```python
from build123d import *

# Parameters (mm, degrees)
SKETCH1_R           = 86.9315
BOSS_EXTRUDE1_DEPTH = 2.54
SKETCH2_W           = 104.14
SKETCH2_H           = 104.14
CUT_EXTRUDE1_DEPTH  = 2.54
SKETCH3_R           = 9.525
SKETCH3_W           = 104.14
SKETCH3_H           = 104.14
CUT_EXTRUDE3_DEPTH  = 203.2


with BuildPart() as part:
    # Sketch1 → Boss-Extrude1 (new body)
    with BuildSketch(Plane(origin=(0, 0, 0), x_dir=(1, 0, 0), z_dir=(0, 1, 0))):
        with Locations(Location((0, 0, 0), (0, 0, 270))):
            Circle(SKETCH1_R)
    extrude(amount=BOSS_EXTRUDE1_DEPTH)

    # Sketch2 → Cut-Extrude1 (cut)
    with BuildSketch(Plane(origin=(0, 2.54, 0), x_dir=(1, 0, 0), z_dir=(0, 1, 0))):
        Rectangle(SKETCH2_W, SKETCH2_H)
    extrude(amount=-CUT_EXTRUDE1_DEPTH, mode=Mode.SUBTRACT)

    # Sketch3 → Cut-Extrude3 (cut)
    with BuildSketch(Plane(origin=(0, 2.54, 0), x_dir=(1, 0, 0), z_dir=(0, 1, 0))):
        with Locations(Location((0, 69.50075, 0), (0, 0, 270))):
            Circle(SKETCH3_R)
        with Locations(Location((69.50075, 0, 0), (0, 0, 270))):
            Circle(SKETCH3_R)
        with Locations(Location((0, -69.50075, 0), (0, 0, 270))):
            Circle(SKETCH3_R)
        with Locations(Location((-69.50075, 0, 0), (0, 0, 270))):
            Circle(SKETCH3_R)
        Rectangle(SKETCH3_W, SKETCH3_H)
    extrude(amount=-CUT_EXTRUDE3_DEPTH, mode=Mode.SUBTRACT)


solid = part.part
```
Can you work these out from the model? Positions are in its coordinate system, mm. Give positions to 0.01 mm unless a question says otherwise; leave off trailing zeros. Loops run counter-clockwise (first coordinate to the right, second up) from the corner with the lowest first, then second, coordinate; pieces in that order, holes last. Notation, with made-up numbers: M 46.5,64.5 L 52.5,64.5 A21 ccw 52.5,92.5 Z; hole C 83.5,64 d1. An arc over 180 degrees is marked long. One line per item, written item: value.
(1) Suppose I cut it at A-A on z = 0. List the corners of the cut face in (x, y) for me, plus the area to 3 significant figures.
Returned:
outline: M -86.93,0 L -79.03,0 L -79.03,2.54 L -86.93,2.54 Z; M -59.98,0 L -52.07,0 L -52.07,2.54 L -59.98,2.54 Z; M 52.07,0 L 59.98,0 L 59.98,2.54 L 52.07,2.54 Z; M 79.03,0 L 86.93,0 L 86.93,2.54 L 79.03,2.54 Z
area: 80.3 mm^2
(2) Suppose I cut it at D-D on z = 18.5. List the corners of the cut face in (x, y) for me.
Returned:
outline: M -84.94,0 L -52.07,0 L -52.07,2.54 L -84.94,2.54 Z; M 52.07,0 L 84.94,0 L 84.94,2.54 L 52.07,2.54 Z
(3) Suppose I cut it at C-C on x = 26.5. List the corners of the cut face in (y, z) for me.
Returned:
outline: M 0,-82.79 L 2.54,-82.79 L 2.54,-52.07 L 0,-52.07 Z; M 0,52.07 L 2.54,52.07 L 2.54,82.79 L 0,82.79 Z
(4) We'd pull the mould along Z, two halves only. Please class faces 1 (the face through (-57, 0, -1)), 2 (the face through (-77.95, 1.29, 4.4)), 3 (the face through (26.112, 1.252, 82.917)): released by +Z, released by -Z, zero draft, split by the parting line, or undercut.
Returned:
face 1: zero draft
face 2: undercut
face 3: split by the parting line
(5) Suppose I cut it at B-B on x = 0. List the corners of the cut face in (y, z) for me, plus the area to 3 significant figures.
Returned:
outline: M 0,-86.93 L 2.54,-86.93 L 2.54,-79.03 L 0,-79.03 Z; M 0,-59.98 L 2.54,-59.98 L 2.54,-52.07 L 0,-52.07 Z; M 0,52.07 L 2.54,52.07 L 2.54,59.98 L 0,59.98 Z; M 0,79.03 L 2.54,79.03 L 2.54,86.93 L 0,86.93 Z
area: 80.3 mm^2
(6) I need wall thicknesses on line 1 (X direction, y = 1.75, z = 0); line 2 (X direction, y = 2, z = 5.5); line 3 (Z direction, x = 73, y = 1.15). Which ranges of each line are inside material? Lowest first, please.
Returned:
line 1: -86.93 to -79.03, -59.98 to -52.07, 52.07 to 59.98, 79.03 to 86.93
line 2: -86.76 to -77.28, -61.72 to -52.07, 52.07 to 61.72, 77.28 to 86.76
line 3: -47.2 to -8.86, 8.86 to 47.2
(7) Will these pins go through, and if not, where does the flat tip stop? pin 1 (15 mm diameter, centred on x = 0, z = 69.5, fed in from +Y); pin 2 (1.3 mm diameter, centred on y = 1.5, z = 24, fed in from -X); pin 3 (0.8 mm diameter, centred on x = 8.5, y = 2, fed in from -Z); pin 4 (1.5 mm diameter, centred on y = 1, z = -39.5, fed in from +X).
Returned:
pin 1: through
pin 2: x = -83.74
pin 3: z = -86.55
pin 4: x = 77.82
